```python
from build123d import *

# Parameters (mm, degrees)
SKETCH151_W     = 65
SKETCH151_H     = 65
SKETCH151_W_2   = 53.065996
SKETCH151_H_2   = 28
POCKET099_DEPTH = 34.001
POCKET100_DEPTH = 22.001
POCKET_DEPTH    = 0.2
CHAMFER_SIZE    = 0.4


with BuildPart() as part:
    # Sketch103 → Revolution002 (revolve)
    with BuildSketch(Plane.YZ):
        Polygon((2.75, 0), (12.5, 0), (12.5, -26), (25.5, -26), (25.5, -34), (2.75, -34), align=None)
    revolve(axis=Axis((0, 0, 0), (0, 0, 1)))

    # Sketch151 (on Face5 of Revolution002) → Pocket099 (cut, through all)
    with BuildSketch(Plane.YX.offset(34)):
        Rectangle(SKETCH151_W, SKETCH151_H)
        Rectangle(SKETCH151_W_2, SKETCH151_H_2, mode=Mode.SUBTRACT)
    extrude(amount=-POCKET099_DEPTH, mode=Mode.SUBTRACT)

    # Sketch142 → Pocket100 (cut, through all)
    with BuildSketch(Plane.XY.offset(-12)):
        Polygon((4.2, 2.424871), (0, 4.849742), (-4.2, 2.424871), (-4.2, -2.424871), (0, -4.849742), (4.2, -2.424871), align=None)
    extrude(amount=-POCKET100_DEPTH, mode=Mode.SUBTRACT)

    # Sketch (on Face4 of Pocket100) → Pocket (cut)
    with BuildSketch(Plane.YX.offset(12)):
        Polygon((0.750555, 4.2), (4.012584, -1.45), (3.262029, -2.75), (-3.262029, -2.75), (-4.012584, -1.45), (-0.750555, 4.2), align=None)
    extrude(amount=-POCKET_DEPTH, mode=Mode.SUBTRACT)

    # Chamfer
    chamfer_edges = [part.edges().sort_by_distance(p)[0] for p in [
        (-7.306329, 24.430873, -34),
        (-14, 0, -34),
        (7.306329, 24.430873, -34),
        (0, -25.5, -34),
        (14, 0, -34),
        (2.1, 3.637307, -34),
        (4.2, 0, -34),
        (2.1, -3.637307, -34),
        (-2.1, -3.637307, -34),
        (-4.2, 0, -34),
        (-2.1, 3.637307, -34),
        (0, -25.5, -26),
        (14, 0, -26),
        (7.306329, 24.430873, -26),
        (-7.306329, 24.430873, -26),
        (-14, 0, -26),
        (14, -21.313141, -30),
        (14, 21.313141, -30),
        (-14, 21.313141, -30),
        (-14, -21.313141, -30),
    ]]
    chamfer(chamfer_edges, length=CHAMFER_SIZE)


with BuildPart() as part_1:
    # Body022019 placement: moved
    add(part.part.moved(Location((0, 92, -72))))


solid = part_1.part
```
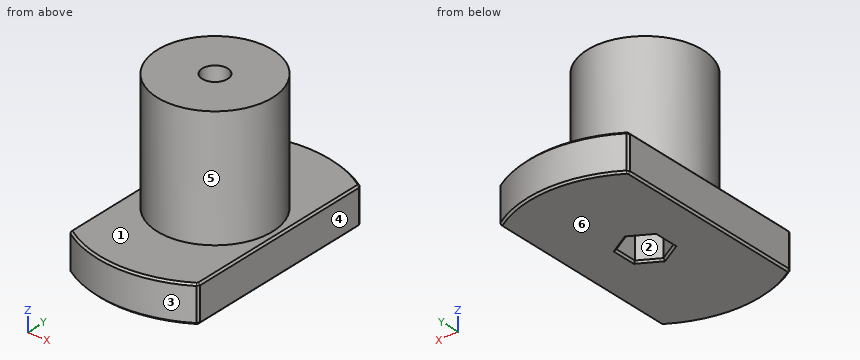
Geometry check sheet. Reference: the model listing, model coordinates, mm. Face numbers are marked on the shaded views. A direction names the side the tool comes from. Round coordinates to 2 decimals unless told otherwise and drop trailing zeros. Order: outer loops, then holes, each group sorted by start corner. A loop starts at its lowest first (then second) coordinate and runs counter-clockwise, first axis right, second up. Notation, with made-up numbers: M 45.5,40 L 79.5,40 A25 cw 79.5,55 Z; hole C 56,4.25 d11. An arc over 180 degrees is marked long. Answer as CSV lines item,"result".
1) Sectioned sample at C-C on z = -82. Record the cut outline in (x, y).
Entries:
outline,"C 0,92 d25; hole C 0,92 d5.5"
2) Gauge pin test, flat ends, axial feed: pin 1 Ø5 at (y, z) = (103, -93.5) entering from -X; pin 2 Ø2 at (x, y) = (0.5, 95.5) entering from -Z; pin 3 Ø1.2 at (x, y) = (-1.5, 89) entering from -Z. Record the tip position at first contact, or that the pin passes through.
Entries:
pin 1,"x = -9.17"
pin 2,"z = -105.68"
pin 3,"z = -83.8"
3) Sectioned sample at D-D on y = 103. Record the cut outline in (x, z).
Entries:
outline,"M -14,-105.6 L -13.6,-106 L 13.6,-106 L 14,-105.6 L 14,-98.4 L 13.6,-98 L 5.94,-98 L 5.94,-72 L -5.94,-72 L -5.94,-98 L -13.6,-98 L -14,-98.4 Z"
4) Sectioned sample at B-B on y = 75. Record the cut outline in (x, z).
Entries:
outline,"M -14,-105.6 L -13.6,-106 L 13.6,-106 L 14,-105.6 L 14,-98.4 L 13.6,-98 L -13.6,-98 L -14,-98.4 Z"
5) Tool access check on the marked faces 5 and 6. Record the directions out of +Z, -Z, +X, -X, +Y, -Y that give a thin tool (end or side, any length) a straight path to the whole face; none if there is none.
Entries:
face 5,"+Z"
face 6,"-Z, +X, -X, +Y, -Y"
6) Thickness scan on probe 1 along X at (y, z) = (92, -80); probe 2 along Y at (x, z) = (0, -74.25); probe 3 along X at (y, z) = (92.5, -92.5). Record the ranges inside material, lowest first. Write a range as [from, to].
Entries:
probe 1,"[-12.5, -2.75], [2.75, 12.5]"
probe 2,"[79.5, 89.25], [94.75, 104.5]"
probe 3,"[-12.49, -4.2], [4.2, 12.49]"
7) Mould release check, pull along X, two halves, no side actions. Record for the marked faces 1, 2, 3 and 4: +X half, -X half, draft (parallel to the pull), parting line (faces both ways), or undercut.
Entries:
face 1,"draft"
face 2,"undercut"
face 3,"parting line"
face 4,"+X half"
8) Sectioned sample at A-A on z = -95.5. Record the cut outline in (x, y).
Entries:
outline,"C 0,92 d25; hole M -4.2,89.58 L 0,87.15 L 4.2,89.58 L 4.2,94.42 L 0,96.85 L -4.2,94.42 Z"
